```python
from build123d import *

# Parameters (mm, degrees)
F0_W     = 101.6
F0_H     = 76.2
F1_DEPTH = 50.8
F2_W     = 96.52
F2_H     = 71.12
F3_DEPTH = 48.26
F4_R     = 6.35
F5_DEPTH = 25.4


with BuildPart() as f1:
    # F0 (on Top) → F1 (new body)
    with BuildSketch(Plane.XY):
        Rectangle(F0_W, F0_H)
    extrude(amount=F1_DEPTH)

    # F2 (on face) → F3 (cut)
    with BuildSketch(Plane.XY.offset(50.8)):
        Rectangle(F2_W, F2_H)
    extrude(amount=-F3_DEPTH, mode=Mode.SUBTRACT)

    # F4 (on face) → F5 (join)
    with BuildSketch(Plane.YZ.offset(50.8)):
        Circle(F4_R)
    extrude(amount=F5_DEPTH)


solid = f1.part
```
The model under review builds one solid part; all positions refer to its coordinate system, in mm. A direction names the side the tool comes from. Round coordinates to 2 decimals unless told otherwise and drop trailing zeros. Loops run counter-clockwise (first coordinate to the right, second up) from the corner with the lowest first, then second, coordinate; pieces in that order, holes last. Notation, with made-up numbers: (-5, 23) - (7, 23) arc R16 cw to (7, 30) - close; hole circle Ø11 at (9, 30.25). An arc over 180 degrees is marked (long way). Write each question's results on one line, items separated by ' | '. Start each with the question number.
Q1. Take a section at C-C on x = -41. Give the boundary of the cut face in (y, z), plus the area to 3 significant figures.
Q2. Take a section at B-B on y = 26. Give the boundary of the cut face in (x, z), plus the area to 3 significant figures.
Q3. Take a section at D-D on y = 0. Give the boundary of the cut face in (x, z).
Q4. Wall thickness on line 1 along Y through (x, z) = (-13, 12); line 2 along X through (y, z) = (5, 3); line 3 along X through (y, z) = (21.5, 47.5): over which ranges is each line inside the solid? List them lowest first. Write a range as [from, to].
Q5. Take a section at A-A on z = 31. Give the boundary of the cut face in (x, y), plus the area to 3 significant figures.
Q6. Insertion check: P1, Ø15, axis at y = 0, z = 15.5, coming from the +X side; P2, Ø3, axis at y = -2.5, z = -3, coming from the -X side; P3, Ø1.5, axis at x = 11, y = 1.5, coming from the -Z side. Each pin has a flat end and moves straight along its axis. Give the tip position at first contact, or say it passes through.
Q7. Draft analysis for pull direction Y (two halves, no side actions). For faces 4 (the flat face through (-1, -35.56, 27)), 5 (the flat face through (76.2, 0, 0)), 6 (the flat face through (-1, 38.1, 25)), state which applies: pulls with the +Y half, pulls with the -Y half, needs draft (parallel to the pull), parting line crosses it, or undercut.
Q8. Tool access review of faces 1 (the flat face through (-1, 35.56, 27)), 2 (the flat face through (50.8, 0, -2)), 3 (the cylindrical face through (63.32, -1.38, -6.2)): name each direction out of +Z, -Z, +X, -X, +Y, -Y from which nothing blocks a thin tool from reaching the whole face with its end or side.
Data:
1) outline: (-38.1, 0) - (38.1, 0) - (38.1, 50.8) - (35.56, 50.8) - (35.56, 2.54) - (-35.56, 2.54) - (-35.56, 50.8) - (-38.1, 50.8) - close | area: 439 mm²
2) outline: (-50.8, 0) - (50.8, 0) - (50.8, 50.8) - (48.26, 50.8) - (48.26, 2.54) - (-48.26, 2.54) - (-48.26, 50.8) - (-50.8, 50.8) - close | area: 503 mm²
3) outline: (-50.8, 0) - (50.8, 0) - (50.8, -6.35) - (76.2, -6.35) - (76.2, 6.35) - (50.8, 6.35) - (50.8, 50.8) - (48.26, 50.8) - (48.26, 2.54) - (-48.26, 2.54) - (-48.26, 50.8) - (-50.8, 50.8) - close
4) line 1: y = [-38.1, -35.56], [35.56, 38.1] | line 2: x = [-50.8, -48.26], [48.26, 76.2] | line 3: x = [-50.8, -48.26], [48.26, 50.8]
5) outline: (-50.8, -38.1) - (50.8, -38.1) - (50.8, 38.1) - (-50.8, 38.1) - close; hole (-48.26, -35.56) - (48.26, -35.56) - (48.26, 35.56) - (-48.26, 35.56) - close | area: 877 mm²
6) P1: stops at x = 50.8 | P2: stops at x = 50.8 | P3: stops at z = 0
7) face 4: undercut | face 5: needs draft | face 6: pulls with the +Y half
8) face 1: +Z | face 2: -Z, -X, +Y, -Y | face 3: +X
